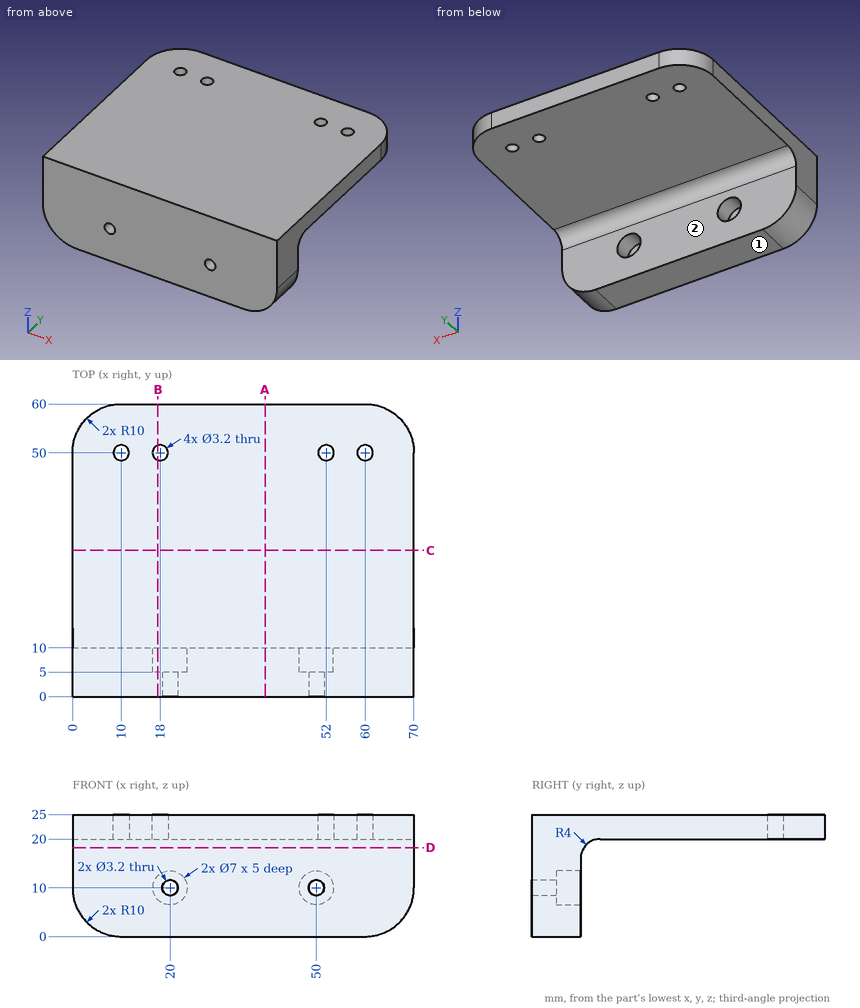
Input: dimensioned drawing with shaded views. Units: mm. Origin: part minimum x, y, z. A direction names the side the tool comes from. Round coordinates to 2 decimals unless told otherwise and drop trailing zeros. Order: outer loops, then holes, each group sorted by start corner. A loop starts at its lowest first (then second) coordinate and runs counter-clockwise, first axis right, second up. Notation, with made-up numbers: (26.25, 60.5) -> (43.25, 60.5) arc R29 cw to (43.25, 98.5) -> close; hole circle Ø9 at (88, 0). An arc over 180 degrees is marked (long way). Put each result on its own line as item: value. Start each with the question number.
Q1. Section D-D on z = 18.25. Return the cut outline in (x, y).
Q2. Line query: probe 1 along X at (y, z) = (6.35, 10); probe 2 along X at (y, z) = (1.8, 10); probe 3 along Y at (x, z) = (18, 23.6). Output: solid intervals per line, ascending.
Q3. First-contact query: pin 1 (3.5 mm diameter, centred on x = 48.5, z = 8.5, fed in from +Y); pin 2 (2 mm diameter, centred on x = 19, z = 16, fed in from +Y); pin 3 (2 mm diameter, centred on x = 21.5, z = 8.5, fed in from +Y). Flat tips, straight axial feed; report the tip coordinate or a pass-through.
Q4. Section B-B on x = 17.5. Return the cut outline in (y, z).
Q5. Section A-A on x = 39.5. Return the cut outline in (y, z), and give its area (3 significant figures).
Q6. Reachability of the marked faces 1 and 2 from +Z, -Z, +X, -X, +Y, -Y: full face, straight path, thin tool, end or side. Return the list, or none.
Q7. Section C-C on y = 30. Return the cut outline in (x, z).
Ans:
1. outline: (0, 0) -> (70, 0) -> (70, 10.69) -> (0, 10.69) -> close
2. probe 1: x = 0 to 16.5, 23.5 to 46.5, 53.5 to 70
2. probe 2: x = 0 to 18.4, 21.6 to 48.4, 51.6 to 70
2. probe 3: y = 0 to 48.4, 51.6 to 60
3. pin 1: stops at y = 10
3. pin 2: stops at y = 10.13
3. pin 3: stops at y = 5
4. outline: (0, 0) -> (10, 0) -> (10, 7.55) -> (5, 7.55) -> (5, 12.45) -> (10, 12.45) -> (10, 16) arc R4 cw to (14, 20) -> (48.48, 20) -> (48.48, 25) -> (0, 25) -> close; (51.52, 20) -> (60, 20) -> (60, 25) -> (51.52, 25) -> close
5. outline: (0, 0) -> (10, 0) -> (10, 16) arc R4 cw to (14, 20) -> (60, 20) -> (60, 25) -> (0, 25) -> close
5. area: 503 mm2
6. face 1: -Z, +X, -X, +Y, -Y
6. face 2: -Z, +X, -X, +Y
7. outline: (0, 20) -> (70, 20) -> (70, 25) -> (0, 25) -> close
